Work out the finished part from the listing and answer in its coordinate system (mm). Face numbers are marked on the shaded views. A direction names the side the tool comes from. Give positions to 0.01 mm unless a question says otherwise; leave off trailing zeros. Order: outer loops, then holes, each group sorted by start corner. A loop starts at its lowest first (then second) coordinate and runs counter-clockwise, first axis right, second up. Notation, with made-up numbers: (13, 24) - (67, 24) arc R17 cw to (67, 32) - close; hole circle Ø8 at (17.5, -38). An arc over 180 degrees is marked (long way). Write each question's results on one line, items separated by ' | '.
from build123d import *

# Parameters (mm, degrees)
SKETCH_1_W                  = 63.5
SKETCH_1_H                  = 63.5
EXTRUDE_1_DEPTH             = 10
HOLE_WIZARD_M31_D           = 3.4
HOLE_WIZARD_M31_CBORE_D     = 6.5
HOLE_WIZARD_M31_CBORE_DEPTH = 3.4
HOLE_WIZARD_M41_D           = 4.5
HOLE_WIZARD_M41_CBORE_D     = 8
HOLE_WIZARD_M41_CBORE_DEPTH = 4.4
SKETCH_8_R                  = 12.5
CUT_EXTRUDE_1_DEPTH         = 7
EXTRUDE_2_DEPTH             = 7
FILLET_1_R                  = 3


with BuildPart() as part:
    # Эскиз1 → Бобышка-Вытянуть1 (new body)
    with BuildSketch(Plane.XY):
        Rectangle(SKETCH_1_W, SKETCH_1_H)
    extrude(amount=EXTRUDE_1_DEPTH)

    # Цековка для винта с внутренним шестигранником M31 (through all)
    with Locations(Plane.XY.offset(10)):
        with Locations((0, 6), (-6, 0), (0, -6), (6, 0)):
            CounterBoreHole(HOLE_WIZARD_M31_D / 2, HOLE_WIZARD_M31_CBORE_D / 2, HOLE_WIZARD_M31_CBORE_DEPTH)

    # Цековка для винта с внутренним шестигранником M41 (through all)
    with Locations(Plane(origin=(0, 0, 0), x_dir=(-1, 0, 0), z_dir=(0, 0, -1))):
        with Locations((-26.75, 26.75), (-26.75, -26.75), (26.75, -26.75), (26.75, 26.75)):
            CounterBoreHole(HOLE_WIZARD_M41_D / 2, HOLE_WIZARD_M41_CBORE_D / 2, HOLE_WIZARD_M41_CBORE_DEPTH)

    # Эскиз8 → Вырез-Вытянуть1 (cut)
    with BuildSketch(Plane(origin=(0, 0, 0), x_dir=(-1, 0, 0), z_dir=(0, 0, -1))):
        with BuildLine():
            Line((-28.75, 16.800125629), (-28.75, -16.800125629))
            ThreePointArc((-28.75, -16.800125629), (-27.974859546, -18.812586809), (-26.05, -19.78508794))
            ThreePointArc((-26.05, -19.78508794), (-21.800252532, -21.800252532), (-19.78508794, -26.05))
            ThreePointArc((-19.78508794, -26.05), (-18.812586809, -27.974859546), (-16.800125629, -28.75))
            Line((-16.800125629, -28.75), (16.800125629, -28.75))
            ThreePointArc((16.800125629, -28.75), (18.812586809, -27.974859546), (19.78508794, -26.05))
            ThreePointArc((19.78508794, -26.05), (21.800252532, -21.800252532), (26.05, -19.78508794))
            ThreePointArc((26.05, -19.78508794), (27.974859546, -18.812586809), (28.75, -16.800125629))
            Line((28.75, -16.800125629), (28.75, 16.800125629))
            ThreePointArc((28.75, 16.800125629), (27.974859546, 18.812586809), (26.05, 19.78508794))
            ThreePointArc((26.05, 19.78508794), (21.800252532, 21.800252532), (19.78508794, 26.05))
            ThreePointArc((19.78508794, 26.05), (18.812586809, 27.974859546), (16.800125629, 28.75))
            Line((16.800125629, 28.75), (-16.800125629, 28.75))
            ThreePointArc((-16.800125629, 28.75), (-18.812586809, 27.974859546), (-19.78508794, 26.05))
            ThreePointArc((-19.78508794, 26.05), (-21.800252532, 21.800252532), (-26.05, 19.78508794))
            ThreePointArc((-26.05, 19.78508794), (-27.974859546, 18.812586809), (-28.75, 16.800125629))
        make_face()
        Circle(SKETCH_8_R, mode=Mode.SUBTRACT)
    extrude(amount=-CUT_EXTRUDE_1_DEPTH, mode=Mode.SUBTRACT)

    # Эскиз9 → Бобышка-Вытянуть2 (add)
    with BuildSketch(Plane(origin=(0, 0, 7), x_dir=(-1, 0, 0), z_dir=(0, 0, -1))):
        with BuildLine():
            Line((20.854569927, 22.97589027), (7.714304216, 9.835624559))
            ThreePointArc((7.714304216, 9.835624559), (8.838834765, 8.838834765), (9.835624559, 7.714304216))
            Line((9.835624559, 7.714304216), (22.97589027, 20.854569927))
            ThreePointArc((22.97589027, 20.854569927), (21.800252532, 21.800252532), (20.854569927, 22.97589027))
        make_face()
        with BuildLine():
            Line((-22.97589027, 20.854569927), (-9.835624559, 7.714304216))
            ThreePointArc((-9.835624559, 7.714304216), (-8.838834765, 8.838834765), (-7.714304216, 9.835624559))
            Line((-7.714304216, 9.835624559), (-20.854569927, 22.97589027))
            ThreePointArc((-20.854569927, 22.97589027), (-21.800252532, 21.800252532), (-22.97589027, 20.854569927))
        make_face()
        with BuildLine():
            Line((7.714304216, -9.835624559), (20.854569927, -22.97589027))
            ThreePointArc((20.854569927, -22.97589027), (21.800252532, -21.800252532), (22.97589027, -20.854569927))
            Line((22.97589027, -20.854569927), (9.835624559, -7.714304216))
            ThreePointArc((9.835624559, -7.714304216), (8.838834765, -8.838834765), (7.714304216, -9.835624559))
        make_face()
        with BuildLine():
            Line((-7.714304216, -9.835624559), (-20.854569927, -22.97589027))
            ThreePointArc((-20.854569927, -22.97589027), (-21.800252532, -21.800252532), (-22.97589027, -20.854569927))
            Line((-22.97589027, -20.854569927), (-9.835624559, -7.714304216))
            ThreePointArc((-9.835624559, -7.714304216), (-8.838834765, -8.838834765), (-7.714304216, -9.835624559))
        make_face()
    extrude(amount=EXTRUDE_2_DEPTH)

    # Скругление1
    fillet_1_edges = [part.edges().sort_by_distance(p)[0] for p in [
        (-20.854569927, 22.97589027, 3.5),
        (-22.97589027, 20.854569927, 3.5),
        (-9.835624559, 7.714304216, 3.5),
        (-7.714304216, 9.835624559, 3.5),
        (9.835624559, -7.714304216, 3.5),
        (7.714304216, -9.835624559, 3.5),
        (20.854569927, -22.97589027, 3.5),
        (22.97589027, -20.854569927, 3.5),
        (22.97589027, 20.854569927, 3.5),
        (20.854569927, 22.97589027, 3.5),
        (7.714304216, 9.835624559, 3.5),
        (9.835624559, 7.714304216, 3.5),
        (-7.714304216, -9.835624559, 3.5),
        (-9.835624559, -7.714304216, 3.5),
        (-22.97589027, -20.854569927, 3.5),
        (-20.854569927, -22.97589027, 3.5),
    ]]
    fillet(fillet_1_edges, radius=FILLET_1_R)


solid = part.part
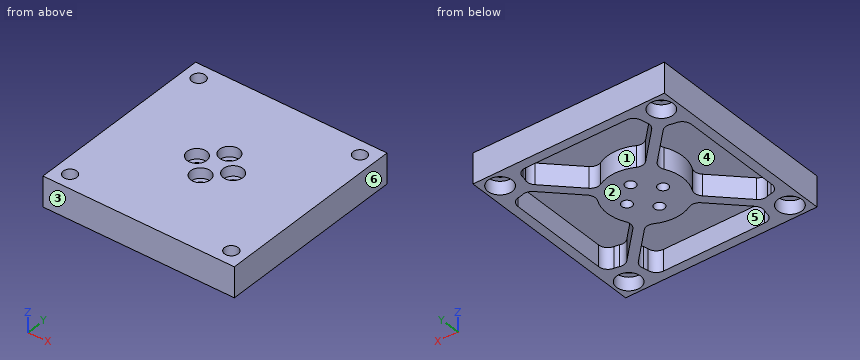
1. A cutting plane is placed at D-D, the plane z = 5.5. State how many separate pieces and enclosed holes the cut face has, then the cut area to 3 significant figures.
Answer list:
separate pieces: 1 | enclosed holes: 12 | area: 1,650 mm^2
2. A tool of negligible diameter and unlimited length cuts with its end or side. For the marked faces 1 and 2, from which of +Z, -Z, +X, -X, +Y, -Y can it reach the whole face along a straight path? Write none if from no direction.
Answer list:
face 1: -Z | face 2: -Z, +X, -X, +Y, -Y
3. Straight lines are drawn through the part: line 1 (Y direction, x = 0, z = 8.65); line 2 (X direction, y = -1.5, z = 9.25); line 3 (X direction, y = -26, z = 7.75). For each, find the intervals that lie inside material, in ascending order. Write a range as [from, to].
Answer list:
line 1: [-31.75, -9.25], [-2.75, 2.75], [9.25, 31.75] | line 2: [-31.75, -8.88], [-3.12, 3.12], [8.88, 31.75] | line 3: [-31.75, -28.87], [-24.63, 24.63], [28.87, 31.75]
4. A cutting plane is placed at C-C, the plane y = -18. Write down the section's boundary in (x, z), then the cut area to 3 significant figures.
Answer list:
outline: (-31.75, 0) - (-28.5, 0) - (-28.5, 7) - (-20.12, 7) - (-20.12, 0) - (-15.88, 0) - (-15.88, 7) - (15.88, 7) - (15.88, 0) - (20.12, 0) - (20.12, 7) - (28.5, 7) - (28.5, 0) - (31.75, 0) - (31.75, 10) - (-31.75, 10) - close | area: 295 mm^2
5. A cutting plane is placed at A-A, the plane y = 0. Write down the section's boundary in (x, z).
Answer list:
outline: (-31.75, 0) - (-28.75, 0) - (-28.75, 7) - (-12.5, 7) - (-12.5, 0) - (-7.7, 0) - (-7.7, 6.6) - (-9.25, 6.6) - (-9.25, 10) - (-31.75, 10) - close; (-4.3, 0) - (4.3, 0) - (4.3, 6.6) - (2.75, 6.6) - (2.75, 10) - (-2.75, 10) - (-2.75, 6.6) - (-4.3, 6.6) - close; (7.7, 0) - (12.5, 0) - (12.5, 7) - (28.75, 7) - (28.75, 0) - (31.75, 0) - (31.75, 10) - (9.25, 10) - (9.25, 6.6) - (7.7, 6.6) - close
6. Determine the mould class of the marked faces 3, 4, 5 and 6 for opening direction X: +X half, -X half, draft (parallel to the pull), parting line (faces both ways), or undercut.
Answer list:
face 3: draft | face 4: undercut | face 5: undercut | face 6: +X half
7. Given P1, Ø4.5, axis at x = 0, y = -6, coming from the +Z side; P2, Ø5, axis at x = 6, y = 1.5, coming from the +Z side; P3, Ø4, axis at x = 27.5, y = 28, coming from the -Z side; P4, Ø9, axis at x = -5.5, y = -21, coming from the -Z side, each flat-ended and moving along its own axis, determine where each tip first touches the part or whether it passes through.
Answer list:
P1: z = 6.6 | P2: z = 10 | P3: z = 4.4 | P4: z = 7
